Geometry check sheet. Reference: the model listing, model coordinates, mm. Give positions to 0.01 mm unless a question says otherwise; leave off trailing zeros. Loops run counter-clockwise (first coordinate to the right, second up) from the corner with the lowest first, then second, coordinate; pieces in that order, holes last.
1. Material ranges on L1, parallel to X at y = 3.2, z = 0; L2, parallel to Z at x = 136, y = -8.5; L3, parallel to Y at x = 139.5, z = 146, recorded low to high.
2. Cross-section at A-A, the plane x = 0. Record the cut outline in (y, z), plus the area to 3 significant figures.
3. Cross-section at C-C, the plane z = 79.5. Record the cut outline in (x, y), plus the area to 3 significant figures.
4. Cross-section at D-D, the plane x = 87. Record the cut outline in (y, z), plus the area to 3 significant figures.
5. Go/stop test with flat-tipped pins: pin 1 Ø4 at (x, z) = (30, 53.5) entering from +Y; pin 2 Ø5 at (x, y) = (84, 8) entering from +Z; pin 3 Ø1.5 at (x, y) = (154.5, 10) entering from -Z; pin 4 Ø1 at (y, z) = (0, 84.5) entering from -X. Record where each tip stops, or that it passes through.
6. Cross-section at B-B, the plane z = 0. Record the cut outline in (x, y).
7. Release check for a two-part mould opening along Z. For faces 1 (the cylindrical face through (4.065, 1.972, -0.534)), 2 (the cylindrical face through (168.281, 16.715, 151.736)), 3 (the cylindrical face through (34.078, 1.972, 33.689)), 4 (the flat face through (-0.82, 1.97, 18.34)) record: +Z half, -Z half, draft (parallel to the pull), parting line (faces both ways), or undercut.
from build123d import *

# Parameters (mm, degrees)
SKETCH_2_R      = 4.1
SKETCH_2_R_2    = 2.1
EXTRUDE_1_DEPTH = 4
FILLET_1_R      = 400
EXTRUDE_4_DEPTH = 30
EXTRUDE_5_REACH = 231.249
SKETCH_8_W      = 30
SKETCH_8_H      = 13
FILLET_5_R      = 1


with BuildPart() as part:
    # 草图2 → 凸台-拉伸1 (new body)
    with BuildSketch(Plane(origin=(0, 0, 0), x_dir=(1, 0, 0), z_dir=(0, 1, 0))):
        with BuildLine():
            Line((136.929210249, -162.385054371), (179.35561712, -162.385054371))
            Line((179.35561712, -162.385054371), (8.485281374, 8.485281374))
            ThreePointArc((8.485281374, 8.485281374), (-7.971171133, 8.969973844), (-9.423568154, -7.429425499))
            Line((-9.423568154, -7.429425499), (22.627416998, -48.083261121))
            Line((22.627416998, -48.083261121), (136.929210249, -162.385054371))
        make_face()
        with Locations(Location((0, 0, 0), (0, 0, 270))):
            Circle(SKETCH_2_R, mode=Mode.SUBTRACT)
        with Locations(Location((35.355339059, -35.355339059, 0), (0, 0, 270))):
            Circle(SKETCH_2_R_2, mode=Mode.SUBTRACT)
    extrude(amount=EXTRUDE_1_DEPTH)

    # 圆角1
    fillet_1_edges = [part.edges().sort_by_distance(p)[0] for p in [
        (22.627416998, 2, 48.083261121),
    ]]
    fillet(fillet_1_edges, radius=FILLET_1_R)

    # 草图6 → 凸台-拉伸4 (add)
    with BuildSketch(Plane(origin=(-12.727922061, 0, 12.727922061), x_dir=(0.7071067811865476, 0, 0.7071067811865475), z_dir=(-0.7071067811865475, 0, 0.7071067811865476))):
        Polygon((191.647146219, 4), (191.647146219, 0), (211.647146219, -13), (211.647146219, 17), align=None)
    extrude(amount=-EXTRUDE_4_DEPTH)

    # 凸台-拉伸5: up to this face of the body (flat: up to its plane)
    extrude_5_end = Plane(part.part.faces().sort_by_distance((158.142413684, 2, 162.385054371))[0])
    # 草图8 → 凸台-拉伸5 (add, up to the picked face)
    with BuildSketch(Plane(origin=(149.65713231, 0, 149.65713231), x_dir=(0.7071067811865475, 0, -0.7071067811865476), z_dir=(0.7071067811865476, 0, 0.7071067811865475)), mode=Mode.PRIVATE) as extrude_5_sk1:
        with Locations((-3, 10.5)):
            Rectangle(SKETCH_8_W, SKETCH_8_H)
    extrude_5_tool1 = split(extrude(extrude_5_sk1.sketch, amount=EXTRUDE_5_REACH, mode=Mode.PRIVATE), bisect_by=extrude_5_end, keep=Keep.BOTH, mode=Mode.PRIVATE)
    # 草图8 → 凸台-拉伸5 (add, up to the picked face)
    with BuildSketch(Plane(origin=(149.65713231, 0, 149.65713231), x_dir=(0.7071067811865475, 0, -0.7071067811865476), z_dir=(0.7071067811865476, 0, 0.7071067811865475)), mode=Mode.PRIVATE) as extrude_5_sk2:
        with Locations((-3, -6.5)):
            Rectangle(SKETCH_8_W, SKETCH_8_H)
    extrude_5_tool2 = split(extrude(extrude_5_sk2.sketch, amount=EXTRUDE_5_REACH, mode=Mode.PRIVATE), bisect_by=extrude_5_end, keep=Keep.BOTH, mode=Mode.PRIVATE)
    add(extrude_5_tool1.solids().sort_by(Axis((147.535812, 10.5, 151.778453), (0.7071067811865476, 0, 0.7071067811865475)))[0])
    add(extrude_5_tool2.solids().sort_by(Axis((147.535812, -6.5, 151.778453), (0.7071067811865476, 0, 0.7071067811865475)))[0])

    # 圆角5
    fillet_5_edges = [part.edges().sort_by_distance(p)[0] for p in [
        (147.535811966, 17, 151.778452653),
        (151.071345872, -6.5, 134.100783124),
        (147.535811966, -13, 151.778452653),
        (151.071345872, 10.5, 134.100783124),
        (168.749015402, 17, 151.778452653),
        (168.749015402, -13, 151.778452653),
        (179.35561712, 2, 162.385054371),
    ]]
    fillet(fillet_5_edges, radius=FILLET_5_R)


solid = part.part
Result:
1. L1: x = -12 to -4.1, 4.1 to 16.97
1. L2: z = 153.52 to 161.46
1. L3: y = -6.65 to 10.65
2. outline: (0, -12) - (4, -12) - (4, -4.1) - (0, -4.1) - close; (0, 4.1) - (4, 4.1) - (4, 19.38) - (0, 19.38) - close
2. area: 92.7 mm2
3. outline: (54.04, 0) - (96.47, 0) - (96.47, 4) - (54.04, 4) - close
3. area: 170 mm2
4. outline: (0, 70.03) - (4, 70.03) - (4, 112.46) - (0, 112.46) - close
4. area: 170 mm2
5. pin 1: stops at y = 4
5. pin 2: passes through
5. pin 3: stops at z = 136.78
5. pin 4: stops at x = 58.54
6. outline: (-12, 0) - (-4.1, 0) - (-4.1, 4) - (-12, 4) - close; (4.1, 0) - (16.97, 0) - (16.97, 4) - (4.1, 4) - close
7. face 1: undercut
7. face 2: -Z half
7. face 3: undercut
7. face 4: +Z half
